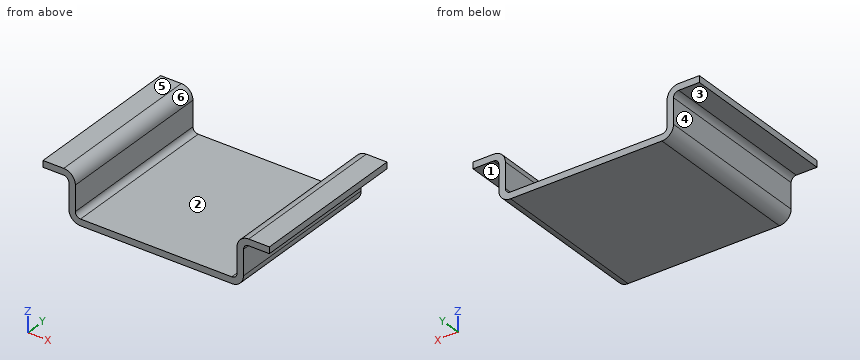
```python
from build123d import *

# Parameters (mm, degrees)
F1_DEPTH = 25


with BuildPart() as f1:
    # F0 (on Front) → F1 (new body)
    with BuildSketch(Plane.XZ):
        with BuildLine():
            Line((-11.7, 0), (0, 0))
            Line((0, 0), (11.7, 0))
            ThreePointArc((11.7, 0), (12.972792, 0.527208), (13.5, 1.8))
            Line((13.5, 1.8), (13.5, 5.7))
            ThreePointArc((13.5, 5.7), (13.734315, 6.265685), (14.3, 6.5))
            Line((14.3, 6.5), (17.5, 6.5))
            Line((17.5, 6.5), (17.5, 7.5))
            Line((17.5, 7.5), (14.3, 7.5))
            ThreePointArc((14.3, 7.5), (13.027208, 6.972792), (12.5, 5.7))
            Line((12.5, 5.7), (12.5, 1.8))
            ThreePointArc((12.5, 1.8), (12.265685, 1.234315), (11.7, 1))
            Line((11.7, 1), (0, 1))
            Line((0, 1), (-11.7, 1))
            ThreePointArc((-11.7, 1), (-12.265685, 1.234315), (-12.5, 1.8))
            Line((-12.5, 1.8), (-12.5, 5.7))
            ThreePointArc((-12.5, 5.7), (-13.027208, 6.972792), (-14.3, 7.5))
            Line((-14.3, 7.5), (-17.5, 7.5))
            Line((-17.5, 7.5), (-17.5, 6.5))
            Line((-17.5, 6.5), (-14.3, 6.5))
            ThreePointArc((-14.3, 6.5), (-13.734315, 6.265685), (-13.5, 5.7))
            Line((-13.5, 5.7), (-13.5, 1.8))
            ThreePointArc((-13.5, 1.8), (-12.972792, 0.527208), (-11.7, 0))
        make_face()
    extrude(amount=F1_DEPTH)


solid = f1.part
```
The listing builds one solid part. Answer for the finished solid, in the listing's coordinates (mm). Face numbers are marked on the shaded views. A direction names the side the tool comes from. Give positions to 0.01 mm unless a question says otherwise; leave off trailing zeros. Order: outer loops, then holes, each group sorted by start corner. A loop starts at its lowest first (then second) coordinate and runs counter-clockwise, first axis right, second up. Notation, with made-up numbers: (-35, 20.5) -> (-11, 20.5) arc R26 ccw to (-11, 42.5) -> close; hole circle Ø2 at (13, 58). An arc over 180 degrees is marked (long way). Answer as CSV lines item,"result". Start each with the question number.
Q1. A cutting plane is placed at A-A (z = 3). Determine the outline of the cut face in (x, y), then the cut area to 3 significant figures.
Q2. A cutting plane is placed at B-B (y = -7.25). Determine the outline of the cut face in (x, z).
Q3. Determine the mould class of the marked faces 4, 5 and 6 for opening direction X: pulls with the +X half, pulls with the -X half, needs draft (parallel to the pull), parting line crosses it, or undercut.
Q4. Given pin 1 (4.5 mm diameter, centred on y = -12, z = 4.5, fed in from -X); pin 2 (3 mm diameter, centred on y = -11.5, z = 4.5, fed in from +X); pin 3 (1 mm diameter, centred on x = -13, y = -5, fed in from +Z); pin 4 (1.2 mm diameter, centred on y = -16, z = 4, fed in from -X), each flat-ended and moving along its own axis, determine where each tip first touches the part or whether it passes through.
Q5. Find the intervals of material crossed by L1, parallel to X at y = -13, z = 5.5; L2, parallel to Z at x = -9, y = -5; L3, parallel to Z at x = 15.5, y = -22.5, in increasing order.
Q6. A cutting plane is placed at C-C (x = 0.5). Determine the outline of the cut face in (y, z), then the cut area to 3 significant figures.
Q7. Which of the six approach directions +Z, -Z, +X, -X, +Y, -Y give full straight-line access (tool end or side, diameter ignored) to the marked faces 1, 2 and 3?
Results found:
1,outline,"(-13.5, -25) -> (-12.5, -25) -> (-12.5, 0) -> (-13.5, 0) -> close; (12.5, -25) -> (13.5, -25) -> (13.5, 0) -> (12.5, 0) -> close"
1,area,"50.0 mm2"
2,outline,"(-17.5, 6.5) -> (-14.3, 6.5) arc R0.8 cw to (-13.5, 5.7) -> (-13.5, 1.8) arc R1.8 ccw to (-11.7, 0) -> (11.7, 0) arc R1.8 ccw to (13.5, 1.8) -> (13.5, 5.7) arc R0.8 cw to (14.3, 6.5) -> (17.5, 6.5) -> (17.5, 7.5) -> (14.3, 7.5) arc R1.8 ccw to (12.5, 5.7) -> (12.5, 1.8) arc R0.8 cw to (11.7, 1) -> (-11.7, 1) arc R0.8 cw to (-12.5, 1.8) -> (-12.5, 5.7) arc R1.8 ccw to (-14.3, 7.5) -> (-17.5, 7.5) -> close"
3,face 4,"pulls with the -X half"
3,face 5,"needs draft"
3,face 6,"undercut"
4,pin 1,"x = -17.5"
4,pin 2,"x = 13.56"
4,pin 3,"z = 7.31"
4,pin 4,"x = -13.5"
5,L1,"-13.5 to -12.5, 12.5 to 13.5"
5,L2,"0 to 1"
5,L3,"6.5 to 7.5"
6,outline,"(-25, 0) -> (0, 0) -> (0, 1) -> (-25, 1) -> close"
6,area,"25.0 mm2"
7,face 1,"-Z, +X, +Y, -Y"
7,face 2,"+Z, +Y, -Y"
7,face 3,"-Z, -X, +Y, -Y"
